Part model, mm, in its own coordinate system. A direction names the side the tool comes from. Round coordinates to 2 decimals unless told otherwise and drop trailing zeros. Loops run counter-clockwise (first coordinate to the right, second up) from the corner with the lowest first, then second, coordinate; pieces in that order, holes last.
Autodesk Inventor part; units mm, degrees
ref_plane "YZ Plane" through (0, 0, 0) normal (1, 0, 0) x (0, 1, 0)
ref_plane "XZ Plane" through (0, 0, 0) normal (0, 1, 0) x (-1, 0, 0)
ref_plane "XY Plane" through (0, 0, 0) normal (0, 0, 1) x (1, 0, 0)
sketch "Sketch1" plane through (0, 0, 0) normal (0, 0, 1) x (1, 0, 0)
  circle A0 centre (0, 0) radius 80
  line L0 (40, 40) -> (-40, 40)
  line L1 (-40, 40) -> (-40, -40)
  line L2 (-40, -40) -> (40, -40)
  line L3 (40, -40) -> (40, 40)
  line L4 (40, 40) -> (-40, -40) construction
  line L5 (-40, 40) -> (40, -40) construction
  circle A1 centre (-62.5, 0) radius 8.5
  circle A2 centre (0, 0) radius 62.5 construction
  circle A3 centre (0, -62.5) radius 8.5
  circle A4 centre (62.5, 0) radius 8.5
  circle A5 centre (0, 62.5) radius 8.5
  dimension "d171" = 125
  dimension "d157" = 160
  dimension "d158" = 80
  dimension "d159" = 80
  dimension "d170" = 17
  dimension "d174" = 360
extrude "Plate5" add sketch "Sketch1" along normal blind 3
chamfer "Corner Chamfer2" distance 20 angle 45 4 edges at (-40, -40, 1.5) (40, -40, 1.5) (-40, 40, 1.5) (40, 40, 1.5)
properties part number "PRS 940-59 FDS MAIN FLANGE" material "Stainless Steel"
1) Wall check: line 1 along Y through (x, z) = (0, 1.4); line 2 along X through (y, z) = (-32.5, 2.1); line 3 along X through (y, z) = (-55.5, 0.45). Give the ranges that are in metal, low to high.
Values:
line 1: y = -80 to -71, -54 to -40, 40 to 54, 71 to 80
line 2: x = -73.1 to -27.5, 27.5 to 73.1
line 3: x = -57.62 to -4.82, 4.82 to 57.62
2) Mould opens along Y. For faces 1 (the face through (34, -34, 3)), 2 (the face through (-71, 0, 1)), 3 (the face through (-17.34, 78.1, 1.48)) say: released by +Y, released by -Y, zero draft, split by the parting line, or undercut.
Values:
face 1: zero draft
face 2: undercut
face 3: split by the parting line
3) Slice it at C-C, the plane x = -33. Give the cut face in (y, z).
Values:
outline: (-72.88, 0) - (-27, 0) - (-27, 3) - (-72.88, 3) - close; (27, 0) - (72.88, 0) - (72.88, 3) - (27, 3) - close
4) Drop flat-ended pins along their axis: pin 1 Ø1.5 at (y, z) = (-8.5, 1.5) entering from -X; pin 2 Ø1.5 at (x, z) = (-1.5, 2) entering from -Y; pin 3 Ø1.5 at (x, z) = (1, 1) entering from +Y. Give the stop position or say it passes through.
Values:
pin 1: stops at x = -79.62
pin 2: stops at y = -80
pin 3: stops at y = 80
5) Slice it at B-B, the plane z = 0.75. Give the cut face in (x, y).
Values:
outline: circle Ø160 at (0, 0); hole circle Ø17 at (-62.5, 0); hole (-40, -20) - (-20, -40) - (20, -40) - (40, -20) - (40, 20) - (20, 40) - (-20, 40) - (-40, 20) - close; hole circle Ø17 at (0, -62.5); hole circle Ø17 at (0, 62.5); hole circle Ø17 at (62.5, 0)
6) Slice it at A-A, the plane y = 0. Give the cut face in (x, z).
Values:
outline: (-80, 0) - (-71, 0) - (-71, 3) - (-80, 3) - close; (-54, 0) - (-40, 0) - (-40, 3) - (-54, 3) - close; (40, 0) - (54, 0) - (54, 3) - (40, 3) - close; (71, 0) - (80, 0) - (80, 3) - (71, 3) - close
7) Tool access for faces 4 (the face through (30, -30, 2)), 5 (the face through (34, -34, 0)): list every direction of +Z, -Z, +X, -X, +Y, -Y with a clear straight run to the whole face (end or side of a thin tool).
Values:
face 4: +Z, -Z
face 5: -Z, +X, -X, +Y, -Y
8) Slice it at D-D, the plane x = -6.5. Give the cut face in (y, z).
Values:
outline: (-79.74, 0) - (-67.98, 0) - (-67.98, 3) - (-79.74, 3) - close; (-57.02, 0) - (-40, 0) - (-40, 3) - (-57.02, 3) - close; (40, 0) - (57.02, 0) - (57.02, 3) - (40, 3) - close; (67.98, 0) - (79.74, 0) - (79.74, 3) - (67.98, 3) - close
